Design review of the part shown in the three views and the two pictorial views. Dimensions are in mm from the part's minimum x, y and z. A direction names the side the tool comes from. Coordinates: 2 decimals unless noted, no trailing zeros. Loops run counter-clockwise (first coordinate to the right, second up) from the corner with the lowest first, then second, coordinate; pieces in that order, holes last. Notation, with made-up numbers: (75, 20) -> (132, 20) arc R29 cw to (132, 50) -> close; hole circle Ø7 at (84, -23). An arc over 180 degrees is marked (long way). Use a Markdown table: item, result. Add a question column.
Q1. For probe 1 along Y at (x, z) = (26, 5.5); probe 2 along Y at (x, z) = (10, 3.25), list the stretches that pass through material, from the lowest coordinate up.
Q2. Take a section at B-B on x = 30.5. Write out the cut boundary in (y, z).
Q3. Take a section at A-A on z = 23.5. Write out the cut boundary in (x, y).
Q4. Clearance check with flat-ended pins moving along their axes: pin 1 Ø5 at (y, z) = (34.5, 14) entering from +X; pin 2 Ø3 at (x, z) = (38.5, 15.5) entering from -Y; pin 3 Ø4 at (y, z) = (9, 12.5) entering from +X. State where each tip first meets the part, or that it passes through.
Q5. For the marked faces 1 and 2, list the 3-axis set-ups (+Z, -Z, +X, -X, +Y, -Y) from which the entire face can be reached by the end or side of a thin tool; tool diameter is ignored.
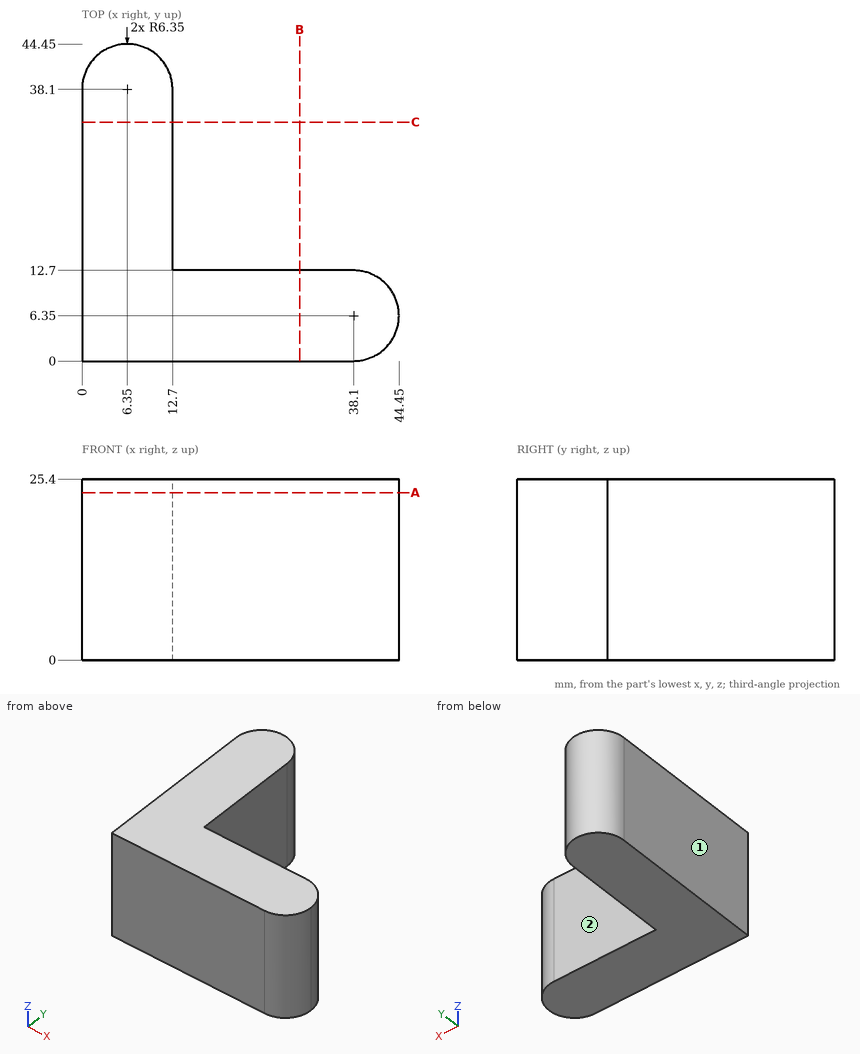
Answer list:
| question | item | result |
|---|---|---|
| 1 | probe 1 | 0 to 12.7 |
| 1 | probe 2 | 0 to 43.3 |
| 2 | outline | (0, 0) -> (12.7, 0) -> (12.7, 25.4) -> (0, 25.4) -> close |
| 3 | outline | (0, 0) -> (38.1, 0) arc R6.35 ccw to (38.1, 12.7) -> (12.7, 12.7) -> (12.7, 38.1) arc R6.35 ccw to (0, 38.1) -> close |
| 4 | pin 1 | x = 12.7 |
| 4 | pin 2 | y = 0 |
| 4 | pin 3 | x = 44.42 |
| 5 | face 1 | +Z, -Z, -X, +Y, -Y |
| 5 | face 2 | +Z, -Z, +X, +Y |
